from build123d import *

# Parameters (mm, degrees)
F1_DEPTH = 9.75
F4_R     = 4
F6_R     = 0.5


with BuildPart() as f1:
    # F0 (on Right) → F1 (new body, symmetric)
    with BuildSketch(Plane.YZ):
        Polygon((4.5580229037, 8.9008104805), (0, 0), (14.5580229037, 3.9008104805), (14.5580229037, 8.9008104805), align=None)
    extrude(amount=F1_DEPTH, both=True)

    # F2 (on face) → F5 section 0
    with BuildSketch(Plane.XY.offset(8.9008104805)):
        Polygon((2.625, 14.1046562736), (-2.625, 14.1046562736), (-5.25, 9.5580229037), (-2.625, 5.0113895339), (2.625, 5.0113895339), (5.25, 9.5580229037), align=None)
    # F4 (on offset) → F5 section 1
    with BuildSketch(Plane.XY.offset(12.9008104805)):
        with Locations((0, 9.5580229037)):
            Circle(F4_R)
    loft()

    # F6
    f6_edges = [f1.edges().sort_by_distance(p)[0] for p in [
        (-9.75, 9.558023, 8.90081),
        (0, 4.558023, 8.90081),
        (9.75, 9.558023, 8.90081),
        (0, 14.558023, 8.90081),
    ]]
    fillet(f6_edges, radius=F6_R)


solid = f1.part
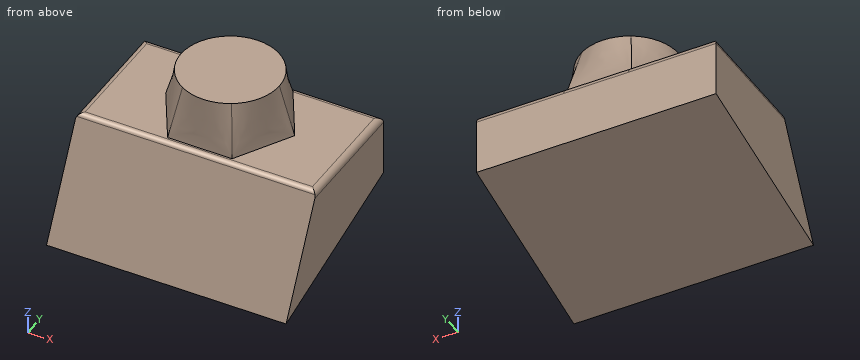
Work out the finished part from the listing and answer in its coordinate system (mm). Give positions to 0.01 mm unless a question says otherwise; leave off trailing zeros. Loops run counter-clockwise (first coordinate to the right, second up) from the corner with the lowest first, then second, coordinate; pieces in that order, holes last. Notation, with made-up numbers: (86.5, 81) -> (113.5, 81) arc R22 cw to (113.5, 108) -> close; hole circle Ø8 at (60.5, 83). An arc over 180 degrees is marked (long way). Use a Markdown table: item, result. Add a question column.
1) The part is cut by section B-B, the plane y = 3. Determine the outline of the cut face in (x, z).
2) Each of these flat-tipped pins is pushed along its axis until it touches: P1, Ø3, axis at x = 7, y = 11, coming from the +Z side; P2, Ø1, axis at x = -5.5, y = 2.5, coming from the -Z side; P3, Ø6, axis at x = 0, z = 7.5, coming from the -Y side. Where does it stop, or does it pass through?
3) The part is cut by section C-C, the plane z = 2. Determine the outline of the cut face in (x, y).
4) The part is cut by section A-A, the plane x = -7.25. Determine the outline of the cut face in (y, z), plus the area to 3 significant figures.
5) Consider line 1 along Y through (x, z) = (6, 8.5); line 2 along Z through (x, y) = (0.25, 7); line 3 along Y through (x, z) = (-4.75, 9.75). Determine where each line is inside the solid, lowest interval first.
Reported:
| question | item | result |
|---|---|---|
| 1 | outline | (-9.75, 0.8) -> (9.75, 0.8) -> (9.75, 5.86) -> (-9.75, 5.86) -> close |
| 2 | P1 | stops at z = 8.9 |
| 2 | P2 | stops at z = 0.54 |
| 2 | P3 | stops at y = 2.3 |
| 3 | outline | (-9.75, 1.02) -> (9.75, 1.02) -> (9.75, 7.46) -> (-9.75, 7.46) -> close |
| 4 | outline | (0, 0) -> (14.56, 3.9) -> (14.56, 8.4) arc R0.5 ccw to (14.06, 8.9) -> (4.86, 8.9) arc R0.5 ccw to (4.42, 8.63) -> close |
| 4 | area | 80.8 mm^2 |
| 5 | line 1 | y = 4.35 to 14.55 |
| 5 | line 2 | z = 1.88 to 12.9 |
| 5 | line 3 | y = 9.06 to 10.05 |
